```python
from build123d import *

# Parameters (mm, degrees)
SKETCH1_R               = 3
BOSS_EXTRUDE1_DEPTH     = 15
SKETCH2_R               = 8.5
BOSS_EXTRUDE2_DEPTH     = 5.25
SKETCH3_R               = 8.5
BOSS_EXTRUDE4_DEPTH     = 31.75
CUT_EXTRUDE4_DEPTH      = 31.75
CUT_EXTRUDE5_REACH      = 42.213
CUT_EXTRUDE5_END_RADIUS = 7.94


with BuildPart() as part:
    # Sketch1 → Boss-Extrude1 (new body)
    with BuildSketch(Plane.XY):
        Circle(SKETCH1_R)
        with BuildLine():
            Line((1.5, 2), (-1.5, 2))
            ThreePointArc((-1.5, 2), (0, -2.5), (1.5, 2))
        make_face(mode=Mode.SUBTRACT)
    extrude(amount=BOSS_EXTRUDE1_DEPTH)

    # Sketch2 → Boss-Extrude2 (add)
    with BuildSketch(Plane(origin=(0, 0, 0), x_dir=(-1, 0, 0), z_dir=(0, 0, -1))):
        with Locations(Location((0, 0, 0), (0, 0, 180))):
            Circle(SKETCH2_R)
    extrude(amount=BOSS_EXTRUDE2_DEPTH)

    # Sketch3 → Boss-Extrude4 (add)
    with BuildSketch(Plane(origin=(0, 0, -5.25), x_dir=(-1, 0, 0), z_dir=(0, 0, -1))):
        with Locations(Location((0, 0, 0), (0, 0, 180))):
            Circle(SKETCH3_R)
    extrude(amount=BOSS_EXTRUDE4_DEPTH)

    # Sketch13 → Cut-Extrude4 (cut)
    with BuildSketch(Plane(origin=(0, 0, -37), x_dir=(-1, 0, 0), z_dir=(0, 0, -1))):
        with BuildLine():
            Line((-2.39, 4.761756731), (-2.39, 7.571756731))
            ThreePointArc((-2.39, 7.571756731), (-4.693985513, -6.403912866), (7.94, 0))
            ThreePointArc((7.94, 0), (6.403912866, 4.693985513), (2.39, 7.571756731))
            Line((2.39, 7.571756731), (2.39, 4.761756731))
            Line((2.39, 4.761756731), (-2.39, 4.761756731))
        make_face()
    extrude(amount=-CUT_EXTRUDE4_DEPTH, mode=Mode.SUBTRACT)

    # Cut-Extrude5: up to this cylinder (the profile starts inside it)
    cut_extrude5_end = Plane(origin=(0, 0, -36.466151), z_dir=(0, 0, -1)) * Cylinder(CUT_EXTRUDE5_END_RADIUS, 101.306, mode=Mode.PRIVATE)
    # Sketch14 → Cut-Extrude5 (cut, up to the surface)
    with BuildSketch(Plane.XZ.offset(-4.761756731), mode=Mode.PRIVATE) as cut_extrude5_sk1:
        with BuildLine():
            Line((2.39, -37), (2.39, -34.61))
            ThreePointArc((2.39, -34.61), (1.689985208, -36.299985206), (3e-09, -37))
            Line((3e-09, -37), (2.39, -37))
        make_face()
    cut_extrude5_tool1 = extrude(cut_extrude5_sk1.sketch, amount=-CUT_EXTRUDE5_REACH, mode=Mode.PRIVATE) & cut_extrude5_end
    add(cut_extrude5_tool1.solids().sort_by_distance((1.856151, 4.761757, -36.466151))[0], mode=Mode.SUBTRACT)
    # Sketch14 → Cut-Extrude5 (cut, up to the surface)
    with BuildSketch(Plane.XZ.offset(-4.761756731), mode=Mode.PRIVATE) as cut_extrude5_sk2:
        with BuildLine():
            ThreePointArc((3e-09, -37), (-1.689985206, -36.299985208), (-2.39, -34.61))
            Line((-2.39, -34.61), (-2.39, -37))
            Line((-2.39, -37), (3e-09, -37))
        make_face()
    cut_extrude5_tool2 = extrude(cut_extrude5_sk2.sketch, amount=-CUT_EXTRUDE5_REACH, mode=Mode.PRIVATE) & cut_extrude5_end
    add(cut_extrude5_tool2.solids().sort_by_distance((-1.856151, 4.761757, -36.466151))[0], mode=Mode.SUBTRACT)


solid = part.part
```
Input: part model. Units: mm. Frame: model coordinates. A direction names the side the tool comes from. Coordinates: 2 decimals unless noted, no trailing zeros. Write each loop counter-clockwise with the first axis right and the second up, starting at its lowest first coordinate (ties: lowest second). Pieces come first, ordered by that corner, then holes. Notation, with made-up numbers: (65.25, -19) -> (87.25, -19) arc R14 cw to (87.25, -2) -> close; hole circle Ø8 at (26, -30.75). An arc over 180 degrees is marked (long way). Answer as a JSON object with one key per item and string values.
1. Access query for faces 4 (the face through (2, -8, -37)), 5 (the face through (-2.39, 6, -20)), 6 (the face through (-0.1, -2.5, 7.4)). Directions: +Z, -Z, +X, -X, +Y, -Y. A direction counts if a zero-diameter tool reaches every point of the face in a straight line with its end or side. Return the directions, or none.
Result set:
{"face 4": "-Z, +X, -X, +Y, -Y", "face 5": "-Z", "face 6": "+Z"}
2. Section A-A on z = -6.5. Return the cut outline in (x, y).
Result set:
{"outline": "circle Ø17 at (0, 0); hole (-2.39, 4.76) -> (-2.39, 7.57) arc R7.94 ccw (long way) to (2.39, 7.57) -> (2.39, 4.76) -> close"}
3. Section D-D on z = -0.5. Return the cut outline in (x, y).
Result set:
{"outline": "circle Ø17 at (0, 0)"}
4. First-contact query: P1, Ø3, axis at x = 0, y = 0, coming from the +Z side; P2, Ø0.9, axis at x = 0, z = 4, coming from the -Y side; P3, Ø4, axis at y = -5.5, z = 1.5, coming from the -X side. Flat tips, straight axial feed; report the tip coordinate or a pass-through.
Result set:
{"P1": "stops at z = 0", "P2": "stops at y = -3", "P3": "stops at x = -7.4"}
5. Section C-C on x = -5.5. Return the cut outline in (y, z).
Result set:
{"outline": "(-6.48, -37) -> (-5.73, -37) -> (-5.73, -5.25) -> (5.73, -5.25) -> (5.73, -37) -> (6.48, -37) -> (6.48, 0) -> (-6.48, 0) -> close"}
6. Mould query, pull axis Y, two halves, no side actions, for faces 1 (the face through (0, 4.762, -21)), 2 (the face through (-1.107, -8.428, -18.241)), 3 (the face through (4, 0, 0)). Classes: released by +Y, released by -Y, zero draft, split by the parting line, or undercut.
Result set:
{"face 1": "undercut", "face 2": "split by the parting line", "face 3": "zero draft"}
7. Section B-B on y = -1. Return the cut outline in (x, z), then the cut area to 3 significant figures.
Result set:
{"outline": "(-8.44, -37) -> (-7.88, -37) -> (-7.88, -5.25) -> (7.88, -5.25) -> (7.88, -37) -> (8.44, -37) -> (8.44, 0) -> (2.83, 0) -> (2.83, 15) -> (2.29, 15) -> (2.29, 0) -> (-2.29, 0) -> (-2.29, 15) -> (-2.83, 15) -> (-2.83, 0) -> (-8.44, 0) -> close", "area": "141 mm2"}
8. Material intervals for line 1 (Y direction, x = 0, z = 6.25); line 2 (X direction, y = 7.25, z = -22); line 3 (Y direction, x = 0, z = -25.5), sorted ascending. Write a range as from..to.
Result set:
{"line 1": "y = -3..-2.5, 2..3", "line 2": "x = -4.44..-3.24, -2.39..2.39, 3.24..4.44", "line 3": "y = -8.5..-7.94, 4.76..8.5"}
